For this review, use the dimensioned drawing (mm, ordinates from the lowest corner) and the shaded views. A direction names the side the tool comes from. Coordinates: 2 decimals unless noted, no trailing zeros. Order: outer loops, then holes, each group sorted by start corner. A loop starts at its lowest first (then second) coordinate and runs counter-clockwise, first axis right, second up. Notation, with made-up numbers: (13, 29.5) -> (62, 29.5) arc R17 cw to (62, 57.5) -> close; hole circle Ø8 at (69.5, 1.5). An arc over 180 degrees is marked (long way). Use one line per item in the form item = value. Start each with the question number.
(1) Take a section at D-D (x = 6). State the section outline as (y, z) points.
(2) Wall thickness on line 1 along Y through (x, z) = (23.39, 10.25); line 2 along Y through (x, z) = (12.5, 10.5); line 3 along X through (y, z) = (43.5, 10.5): over which ranges is each line inside the solid? List them lowest first.
(3) Take a section at A-A (x = 23.39). State the section outline as (y, z) points, then the cut area to 3 significant figures.
(4) Take a section at C-C (z = 7.25). State the section outline as (x, y) points.
(5) Insertion check: pin 1 Ø4.5 at (x, z) = (17, 11) entering from +Y. The pin has a flat end and moves straight along its axis. Give the tip position at first contact, or say it passes through.
(6) Mouldability with a two-part tool opening along X and no side actions: class the marked faces 3, 4, 5 and 6 as +X half, -X half, draft (parallel to the pull), parting line (faces both ways), or undercut.
(7) Take a section at B-B (y = 17). State the section outline as (x, z) points, then the cut area to 3 significant figures.
(8) For the marked faces 1 and 2, list the 3-axis set-ups (+Z, -Z, +X, -X, +Y, -Y) from which the entire face can be reached by the end or side of a thin tool; tool diameter is ignored.
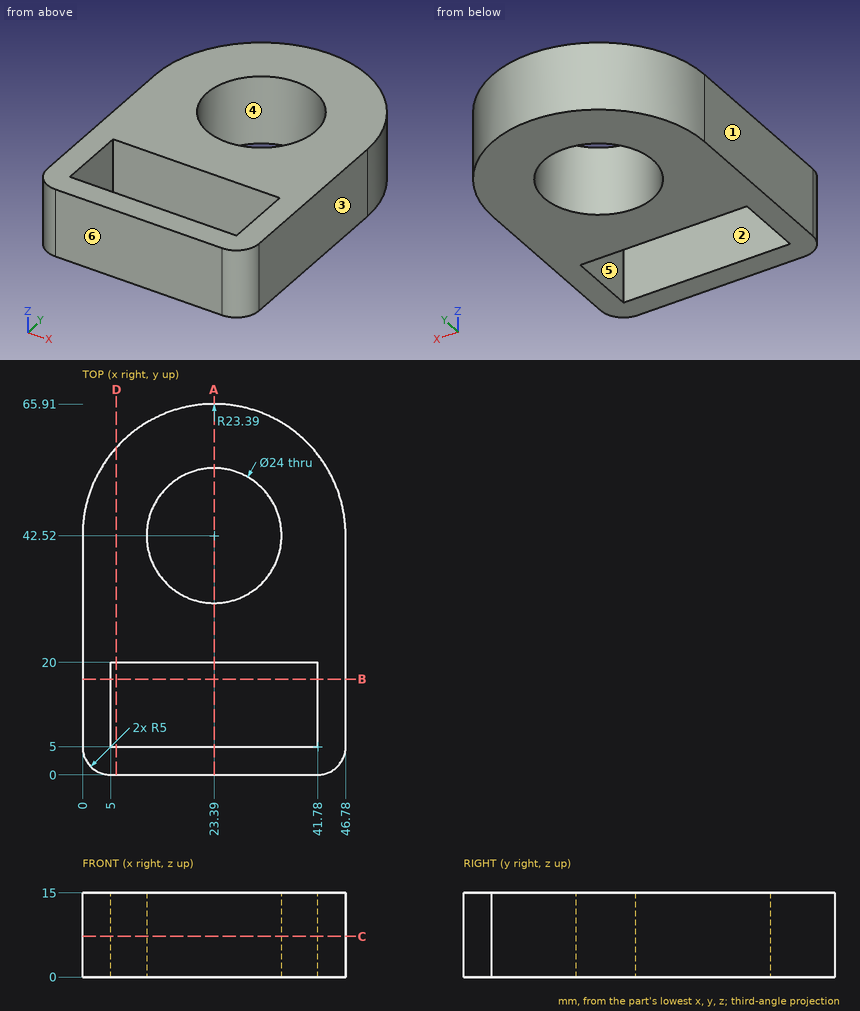
Findings:
q1.outline = (0, 0) -> (5, 0) -> (5, 15) -> (0, 15) -> close; (20, 0) -> (58.16, 0) -> (58.16, 15) -> (20, 15) -> close
q2.line_1 = 0 to 5, 20 to 30.52, 54.52 to 65.91
q2.line_2 = 0 to 5, 20 to 37.48, 47.56 to 63.22
q2.line_3 = 0.02 to 11.43, 35.35 to 46.76
q3.outline = (0, 0) -> (5, 0) -> (5, 15) -> (0, 15) -> close; (20, 0) -> (30.52, 0) -> (30.52, 15) -> (20, 15) -> close; (54.52, 0) -> (65.91, 0) -> (65.91, 15) -> (54.52, 15) -> close
q3.area = 404 mm²
q4.outline = (0, 5) arc R5 ccw to (5, 0) -> (41.78, 0) arc R5 ccw to (46.78, 5.02) -> (46.78, 42.52) arc R23.39 ccw to (0, 42.52) -> close; hole (5, 5) -> (41.78, 5) -> (41.78, 20) -> (5, 20) -> close; hole circle Ø24 at (23.39, 42.52)
q5.pin_1 = 65.54
q6.face_3 = +X half
q6.face_4 = undercut
q6.face_5 = undercut
q6.face_6 = draft
q7.outline = (0, 0) -> (5, 0) -> (5, 15) -> (0, 15) -> close; (41.78, 0) -> (46.78, 0) -> (46.78, 15) -> (41.78, 15) -> close
q7.area = 150 mm²
q8.face_1 = +Z, -Z, -X, +Y, -Y
q8.face_2 = +Z, -Z
